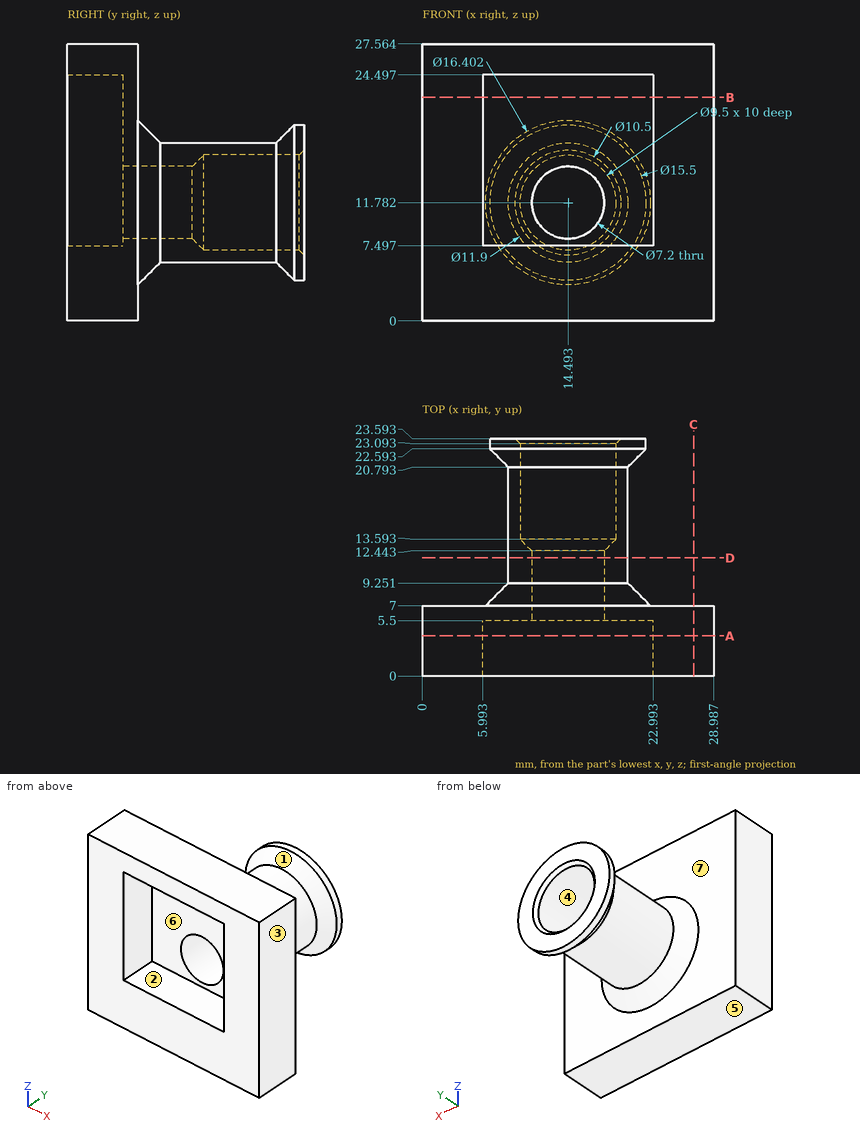
Input: dimensioned drawing with shaded views. Units: mm. Origin: part minimum x, y, z. A direction names the side the tool comes from. Give positions to 0.01 mm unless a question says otherwise; leave off trailing zeros. Order: outer loops, then holes, each group sorted by start corner. A loop starts at its lowest first (then second) coordinate and runs counter-clockwise, first axis right, second up. Notation, with made-up numbers: (-25, -27.5) -> (16, -27.5) arc R14 ccw to (16, -1.5) -> close; hole circle Ø2 at (-28.75, 58.5). An arc over 180 degrees is marked (long way). Answer as a JSON object with one key per item and string values.
Q1. Access query for the marked faces 1, 2 and 3. Directions: +Z, -Z, +X, -X, +Y, -Y. A direction counts if a zero-diameter tool reaches every point of the face in a straight line with its end or side. Return the directions, or none.
Entries:
{"face 1": "none", "face 2": "-Y", "face 3": "+Z, -Z, +X, +Y, -Y"}
Q2. Section D-D (y = 11.75). Output: boundary loops of the cut face in (x, z).
Entries:
{"outline": "circle Ø11.9 at (14.49, 11.78); hole circle Ø7.2 at (14.49, 11.78)"}
Q3. Section C-C (x = 27). Output: boundary loops of the cut face in (y, z).
Entries:
{"outline": "(0, 0) -> (7, 0) -> (7, 27.56) -> (0, 27.56) -> close"}
Q4. Section A-A (y = 4). Output: boundary loops of the cut face in (x, z), plus the area to 3 significant figures.
Entries:
{"outline": "(0, 0) -> (28.99, 0) -> (28.99, 27.56) -> (0, 27.56) -> close; hole (5.99, 7.5) -> (22.99, 7.5) -> (22.99, 24.5) -> (5.99, 24.5) -> close", "area": "510 mm^2"}
Q5. First-contact query: pin 1 (13.5 mm diameter, centred on x = 14.5, z = 15.5, fed in from -Y); pin 2 (3 mm diameter, centred on x = 21, y = 9.5, fed in from -Z) (1 decimal); pin 3 (8.5 mm diameter, centred on x = 14.49, z = 11.78, fed in from +Y); pin 4 (4.5 mm diameter, centred on x = 14.49, z = 11.78, fed in from -Y). Flat tips, straight axial feed; report the tip coordinate or a pass-through.
Entries:
{"pin 1": "stops at y = 5.5", "pin 2": "stops at z = 7.8", "pin 3": "stops at y = 13.1", "pin 4": "passes through"}
Q6. Material intervals for probe 1 along Z at (x, y) = (8.25, 5); probe 2 along Y at (x, z) = (23.5, 22.75); probe 3 along Y at (x, z) = (19.5, 22.5), sorted ascending.
Entries:
{"probe 1": "z = 0 to 7.5, 24.5 to 27.56", "probe 2": "y = 0 to 7", "probe 3": "y = 5.5 to 7"}
Q7. Section B-B (z = 22.25). Output: boundary loops of the cut face in (x, y), plus the area to 3 significant figures.
Entries:
{"outline": "(0, 0) -> (5.99, 0) -> (5.99, 5.5) -> (22.99, 5.5) -> (22.99, 0) -> (28.99, 0) -> (28.99, 7) -> (0, 7) -> close", "area": "109 mm^2"}
Q8. Draft query along Z for the marked faces 4, 5, 6 and 7. Return one class per face: released by +Z, released by -Z, zero draft, split by the parting line, or undercut.
Entries:
{"face 4": "undercut", "face 5": "released by -Z", "face 6": "undercut", "face 7": "zero draft"}
